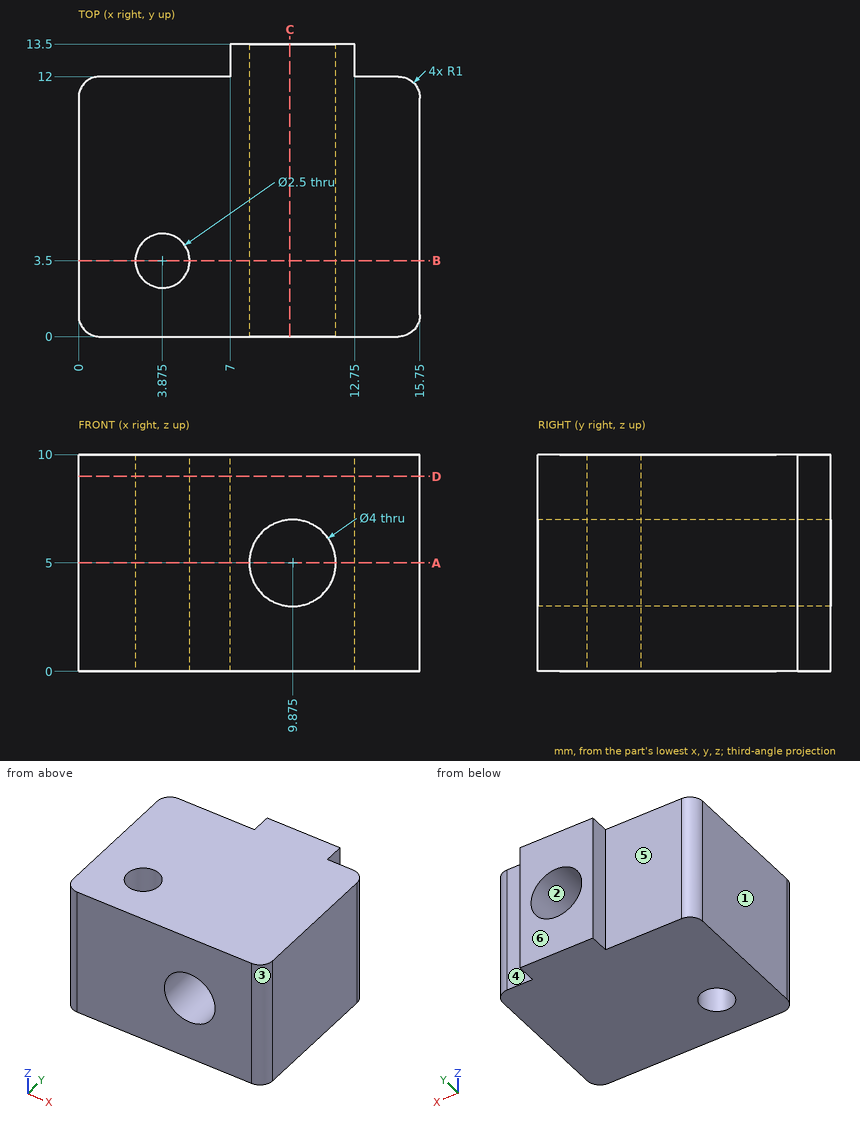
Part print with two shaded views. Sizes in mm from the minimum x, y, z corner. A direction names the side the tool comes from. Round coordinates to 2 decimals unless told otherwise and drop trailing zeros. Order: outer loops, then holes, each group sorted by start corner. A loop starts at its lowest first (then second) coordinate and runs counter-clockwise, first axis right, second up. Notation, with made-up numbers: (36, 47) -> (90, 47) arc R28 ccw to (90, 73) -> close; hole circle Ø5 at (-27.75, 59). An arc over 180 degrees is marked (long way). One line per question, with ' | ' between items.
Q1. Slice it at A-A (z = 5). Write the cut outline in (x, y) (3 decimals), then the cut area to 3 significant figures.
Completed:
outline: (0, 1) arc R1 ccw to (1, 0) -> (7.875, 0) -> (7.875, 13.5) -> (7, 13.5) -> (7, 12) -> (1, 12) arc R1 ccw to (0, 11) -> close; (11.875, 0) -> (14.75, 0) arc R1 ccw to (15.75, 1) -> (15.75, 11) arc R1 ccw to (14.75, 12) -> (12.75, 12) -> (12.75, 13.5) -> (11.875, 13.5) -> close; hole circle Ø2.5 at (3.875, 3.5) | area: 138 mm^2
Q2. Two-plate mould, pull along X, no slides. Class the marked faces 1, 2 and 3: released by +X, released by -X, zero draft, split by the parting line, or undercut.
Completed:
face 1: released by -X | face 2: undercut | face 3: released by +X
Q3. Which spindle directions (+Z, -Z, +X, -X, +Y, -Y) get a long thin tool onto all of the face, cutting with end or side? Do the marked faces 4, 5 and 6. Say none if no direction does.
Completed:
face 4: +Z, -Z, +X, +Y | face 5: +Z, -Z, -X, +Y | face 6: +Z, -Z, +X, -X, +Y
Q4. Probe probe 1 along Y at (x, z) = (4.25, 6.25); probe 2 along X at (y, z) = (3, 5.25); probe 3 along Z at (x, y) = (9.5, 11.5). List the from-to ranges inside material, lowest first.
Completed:
probe 1: y = 0 to 2.31, 4.69 to 12 | probe 2: x = 0 to 2.73, 5.02 to 7.89, 11.86 to 15.75 | probe 3: z = 0 to 3.04, 6.96 to 10
Q5. Slice it at B-B (y = 3.5). Write the cut outline in (x, z) (3 decimals), then the cut area to 3 significant figures.
Completed:
outline: (0, 0) -> (2.625, 0) -> (2.625, 10) -> (0, 10) -> close; (5.125, 0) -> (15.75, 0) -> (15.75, 10) -> (5.125, 10) -> close; hole circle Ø4 at (9.875, 5) | area: 120 mm^2
Q6. Slice it at D-D (z = 9). Write the cut outline in (x, y) (3 decimals), then the cut area to 3 significant figures.
Completed:
outline: (0, 1) arc R1 ccw to (1, 0) -> (14.75, 0) arc R1 ccw to (15.75, 1) -> (15.75, 11) arc R1 ccw to (14.75, 12) -> (12.75, 12) -> (12.75, 13.5) -> (7, 13.5) -> (7, 12) -> (1, 12) arc R1 ccw to (0, 11) -> close; hole circle Ø2.5 at (3.875, 3.5) | area: 192 mm^2
Q7. Slice it at C-C (x = 9.75). Write the cut outline in (y, z), then the cut area to 3 significant figures.
Completed:
outline: (0, 0) -> (13.5, 0) -> (13.5, 3) -> (0, 3) -> close; (0, 7) -> (13.5, 7) -> (13.5, 10) -> (0, 10) -> close | area: 81.1 mm^2
Q8. Drop flat-ended pins along their axis: pin 1 (2.5 mm diameter, centred on x = 9.875, z = 5, fed in from -Y); pin 2 (0.6 mm diameter, centred on x = 13.5, z = 4, fed in from +Y); pin 3 (1.2 mm diameter, centred on y = 13, z = 7, fed in from +X); pin 4 (0.8 mm diameter, centred on y = 13, z = 5.5, fed in from -X). Give the stop position or say it passes through.
Completed:
pin 1: passes through | pin 2: stops at y = 12 | pin 3: stops at x = 12.75 | pin 4: stops at x = 7
